Could you check a few things on this model? Use its own coordinates, in mm. A direction names the side the tool comes from. Coordinates: 2 decimals unless noted, no trailing zeros. Loops run counter-clockwise (first coordinate to the right, second up) from the corner with the lowest first, then second, coordinate; pieces in that order, holes last. Notation, with made-up numbers: (45, -22.5) -> (77, -22.5) arc R31 cw to (77, 3.5) -> close; hole circle Ø11 at (33, 9.25). An arc over 180 degrees is marked (long way). One line per question, with ' | ' between items.
Solid Edge part; units mm, degrees
sketch "Sketch1" plane through (0, 0, 0) normal (0, 0, 1) x (1, 0, 0)
  line L0 (21.15, -21.15) -> (21.15, 21.15)
  line L1 (21.15, 21.15) -> (-21.15, 21.15)
  line L2 (-21.15, 21.15) -> (-21.15, -21.15)
  line L3 (-21.15, -21.15) -> (21.15, -21.15)
extrude "Protrusion1" add sketch "Sketch1" along normal blind 40
sketch "Sketch2" plane through (0, 0, 0) normal (0, 0, 1) x (1, 0, 0)
  circle A0 centre (0, 0) radius 11
extrude "ExtrudedProtrusion_2" add sketch "Sketch2" against normal blind 2
sketch "Sketch3" plane through (0, 0, 0) normal (0, 0, 1) x (1, 0, 0)
  circle A0 centre (0, 0) radius 2.5
extrude "ExtrudedProtrusion_3" add sketch "Sketch3" against normal blind 24
sketch "Sketch4" plane through (0, 0, 0) normal (0, 0, 1) x (1, 0, 0)
  circle A0 centre (15.5, 15.5) radius 1.5
  circle A1 centre (-15.5, 15.5) radius 1.5
  circle A2 centre (-15.5, -15.5) radius 1.5
  circle A3 centre (15.5, -15.5) radius 1.5
extrude "ExtrudedCutout_1" cut sketch "Sketch4" along normal blind 4.5
chamfer "Chamfer_1" distance 5 angle 45 4 edges at (21.15, 21.15, 20) (-21.15, 21.15, 20) (-21.15, -21.15, 20) (21.15, -21.15, 20)
fillet "Round_1" radius 1 8 edges at (0, 21.15, 40) (-18.65, 18.65, 40) (-21.15, 0, 40) (-18.65, -18.65, 40) (0, -21.15, 40) (18.65, -18.65, 40) (21.15, 0, 40) (18.65, 18.65, 40)
chamfer "Chamfer_2" distance 0.5 angle 45 1 edges at (-2.5, 0, -24)
Q1. Imagine slicing it at A-A on x = 0. Write out the boundary of the cut face in (y, z).
Values follow:
outline: (-21.15, 0) -> (-11, 0) -> (-11, -2) -> (-2.5, -2) -> (-2.5, -23.5) -> (-2, -24) -> (2, -24) -> (2.5, -23.5) -> (2.5, -2) -> (11, -2) -> (11, 0) -> (21.15, 0) -> (21.15, 39) arc R1 ccw to (20.15, 40) -> (-20.15, 40) arc R1 ccw to (-21.15, 39) -> close
Q2. Please list where these lines run through material, in increasing order: L1, parallel to Y at x = -15.5, z = 1.9; L2, parallel to Y at x = 15, z = 1; L3, parallel to Z at x = 4, y = 10. Write a range as [from, to].
Values follow:
L1: y = [-21.15, -17], [-14, 14], [17, 21.15] | L2: y = [-21.15, -16.91], [-14.09, 14.09], [16.91, 21.15] | L3: z = [-2, 40]
Q3. Imagine slicing it at C-C on z = 21. Write out the boundary of the cut face in (x, y), plus the area to 3 significant figures.
Values follow:
outline: (-21.15, -16.15) -> (-16.15, -21.15) -> (16.15, -21.15) -> (21.15, -16.15) -> (21.15, 16.15) -> (16.15, 21.15) -> (-16.15, 21.15) -> (-21.15, 16.15) -> close | area: 1,740 mm2
Q4. For faces 4 (the face through (0, 0, -24)), 5 (the face through (-16, -15, 4.5)), which set-ups out of +Z, -Z, +X, -X, +Y, -Y let a thin tool reach every point of the face, with its end or its side?
Values follow:
face 4: -Z, +X, -X, +Y, -Y | face 5: -Z
Q5. Imagine slicing it at D-D on x = -12. Write out the boundary of the cut face in (y, z), plus the area to 3 significant figures.
Values follow:
outline: (-21.15, 0) -> (21.15, 0) -> (21.15, 39) arc R1 ccw to (20.15, 40) -> (-20.15, 40) arc R1 ccw to (-21.15, 39) -> close | area: 1,690 mm2
Q6. For pin 1 (1.5 mm diameter, centred on x = 15.5, y = -16, fed in from -Z); pin 2 (2.5 mm diameter, centred on x = 16, y = 15.5, fed in from -Z); pin 3 (12 mm diameter, centred on x = -9.5, y = 12, fed in from -Z); pin 4 (11 mm diameter, centred on x = 2, y = 5, fed in from -Z), each with a flat end and sliding along its axis, tell me the tip position at first contact or that it passes through.
Values follow:
pin 1: stops at z = 4.5 | pin 2: stops at z = 0 | pin 3: stops at z = -2 | pin 4: stops at z = -24
Q7. We'd pull the mould along X, two halves only. Please class faces 1 (the face through (0, 0, 40)), 2 (the face through (-16, 16, 4.5)), 3 (the face through (-2.38, -10.74, -0.99)): released by +X, released by -X, zero draft, split by the parting line, or undercut.
Values follow:
face 1: zero draft | face 2: undercut | face 3: split by the parting line
